Design review of the part built by this model. Coordinates are the model's own, in mm. Coordinates: 2 decimals unless noted, no trailing zeros. Loops run counter-clockwise (first coordinate to the right, second up) from the corner with the lowest first, then second, coordinate; pieces in that order, holes last. Notation, with made-up numbers: (10, 85.25) - (34, 85.25) arc R22 cw to (34, 109.25) - close; hole circle Ø8 at (10.5, 32). An arc over 180 degrees is marked (long way). Answer in a Markdown table with one row per item. Add a question column.
(1) We need section D-D, the plane x = 9.5. Write out the cut boundary in (y, z).
(2) The part is to be moulded in two halves that separate along X. For faces 1 (the face through (0, 0, 0)), 2 (the face through (-30, 0, 0)), 3 (the face through (0, -14, 3)), say which applies: released by +X, released by -X, zero draft, split by the parting line, or undercut.
(3) We need section C-C, the plane x = 0. Write out the cut boundary in (y, z).
(4) We need section B-B, the plane y = -0.75. Write out the cut boundary in (x, z).
(5) We need section A-A, the plane z = -3.75. Write out the cut boundary in (x, y), plus the area to 3 significant figures.
(6) To check wall thickness, follow L1, parallel to X at y = -7.25, z = -2; L2, parallel to X at y = 6, z = -7.5; L3, parallel to Z at x = 3.5, y = -5. State the ranges of each line that lie inside material, in increasing order. Write a range as [from, to].
from build123d import *

# Parameters (mm, degrees)
F0_W     = 60
F0_H     = 28
F1_DEPTH = 14
F2_R     = 14
F3_DEPTH = 50


with BuildPart() as f1:
    # F0 (on Top) → F1 (new body, symmetric)
    with BuildSketch(Plane.XY):
        Rectangle(F0_W, F0_H)
    extrude(amount=F1_DEPTH, both=True)

    # F2 (on Front) → F3 (cut, symmetric)
    with BuildSketch(Plane.XZ):
        with Locations((0, -14)):
            Circle(F2_R)
    extrude(amount=F3_DEPTH, both=True, mode=Mode.SUBTRACT)


solid = f1.part
Responses:
| question | item | result |
|---|---|---|
| 1 | outline | (-14, -3.72) - (14, -3.72) - (14, 14) - (-14, 14) - close |
| 2 | face 1 | undercut |
| 2 | face 2 | released by -X |
| 2 | face 3 | zero draft |
| 3 | outline | (-14, 0) - (14, 0) - (14, 14) - (-14, 14) - close |
| 4 | outline | (-30, -14) - (-14, -14) arc R14 cw to (14, -14) - (30, -14) - (30, 14) - (-30, 14) - close |
| 5 | outline | (-30, -14) - (-9.54, -14) - (-9.54, 14) - (-30, 14) - close; (9.54, -14) - (30, -14) - (30, 14) - (9.54, 14) - close |
| 5 | area | 1,150 mm2 |
| 6 | L1 | x = [-30, -7.21], [7.21, 30] |
| 6 | L2 | x = [-30, -12.4], [12.4, 30] |
| 6 | L3 | z = [-0.44, 14] |
